```python
from build123d import *

# Parameters (mm, degrees)
F1_DEPTH = 200
F2_R     = 2
F4_DEPTH = 2


with BuildPart() as f1:
    # F0 (on Front) → F1 (new body)
    with BuildSketch(Plane.XZ):
        Polygon((35, 0), (0, 0), (0, -345), (28, -345), (28, -295), (8, -271.164928), (8, -191.164928), (30, -130.720425), (30, -80.720425), (28, -80.720425), (28, -130.367771), (6, -190.812274), (6, -271.892869), (26, -295.72794), (26, -343), (2, -343), (2, -2), (33, -2), (33, -23), (35, -23), align=None)
    extrude(amount=F1_DEPTH)

    # F2
    f2_edges = [f1.edges().sort_by_distance(p)[0] for p in [
        (0, -100, 0),
        (35, -100, 0),
        (33, -100, -2),
        (2, -100, -2),
        (0, -100, -345),
        (2, -100, -343),
        (28, -100, -345),
        (26, -100, -343),
        (26, -100, -295.72794),
        (28, -100, -295),
        (8, -100, -271.164928),
        (6, -100, -271.892869),
        (6, -100, -190.812274),
        (8, -100, -191.164928),
        (30, -100, -130.720425),
        (28, -100, -130.367771),
    ]]
    fillet(f2_edges, radius=F2_R)

    # F3 (on face) → F4 (cut)
    with BuildSketch(Plane(origin=(0, 0, 0), x_dir=(0, -1, 0), z_dir=(-1, 0, 0))):
        with BuildLine():
            Line((70, -50), (30, -50))
            ThreePointArc((30, -50), (26.464466, -51.464466), (25, -55))
            Line((25, -55), (25, -290))
            ThreePointArc((25, -290), (26.464466, -293.535534), (30, -295))
            Line((30, -295), (70, -295))
            ThreePointArc((70, -295), (73.535534, -293.535534), (75, -290))
            Line((75, -290), (75, -55))
            ThreePointArc((75, -55), (73.535534, -51.464466), (70, -50))
        make_face()
        with BuildLine():
            ThreePointArc((175, -55), (173.535534, -51.464466), (170, -50))
            Line((170, -50), (130, -50))
            ThreePointArc((130, -50), (126.464466, -51.464466), (125, -55))
            Line((125, -55), (125, -290))
            ThreePointArc((125, -290), (126.464466, -293.535534), (130, -295))
            Line((130, -295), (170, -295))
            ThreePointArc((170, -295), (173.535534, -293.535534), (175, -290))
            Line((175, -290), (175, -55))
        make_face()
    extrude(amount=-F4_DEPTH, mode=Mode.SUBTRACT)


solid = f1.part
```
Source: CAD feature listing. Evaluate the final solid. Frame: model axes, mm. A direction names the side the tool comes from. Give positions to 0.01 mm unless a question says otherwise; leave off trailing zeros. Order: outer loops, then holes, each group sorted by start corner. A loop starts at its lowest first (then second) coordinate and runs counter-clockwise, first axis right, second up. Notation, with made-up numbers: (-37.5, -13) -> (14.5, -13) arc R37 ccw to (14.5, 24) -> close; hole circle Ø8 at (76.5, 9). An arc over 180 degrees is marked (long way). Use a Markdown table: item, result.
Q1. Section A-A (z = -205). Return the cut outline in (x, y), and give its area (3 significant figures).
A:
| item | result |
|---|---|
| outline | (0, -200) -> (2, -200) -> (2, -175) -> (0, -175) -> close; (0, -125) -> (2, -125) -> (2, -75) -> (0, -75) -> close; (0, -25) -> (2, -25) -> (2, 0) -> (0, 0) -> close; (6, -200) -> (8, -200) -> (8, 0) -> (6, 0) -> close |
| area | 600 mm^2 |
Q2. Material intervals for line 1 (X direction, y = -166, z = -14.5); line 2 (X direction, y = -159, z = -191.5); line 3 (Z direction, x = 3.5, y = -19), sorted ascending. Write a range as [from, to].
A:
| item | result |
|---|---|
| line 1 | [0, 2], [33, 35] |
| line 2 | [6, 8] |
| line 3 | [-345, -342.94], [-2.06, 0] |
Q3. Pull-direction query (X, two-part tool) for faces 1 (the face through (0, -99, -170)), 2 (the face through (26, -99, -318)), 3 (the face through (14, -99, -345)); classes: +X half, -X half, draft (parallel to the pull), parting line (faces both ways), or undercut.
A:
| item | result |
|---|---|
| face 1 | -X half |
| face 2 | undercut |
| face 3 | draft |
Q4. First-contact query: P1, Ø1.6, axis at x = 1, y = -50, coming from the +Z side; P2, Ø1, axis at x = 1, y = -145, coming from the -Z side; P3, Ø4, axis at x = 4.5, z = -158, coming from the +Y side; P4, Ø23.5, axis at y = -84, z = -318, coming from the +X side. Flat tips, straight axial feed; report the tip coordinate or a pass-through.
A:
| item | result |
|---|---|
| P1 | z = -0.01 |
| P2 | z = -344.94 |
| P3 | through |
| P4 | x = 28 |
Q5. Section B-B (x = 15.5). Return the cut outline in (y, z), and give its area (3 significant figures).
A:
| item | result |
|---|---|
| outline | (-200, -345) -> (0, -345) -> (0, -343) -> (-200, -343) -> close; (-200, -283.21) -> (0, -283.21) -> (0, -280.1) -> (-200, -280.1) -> close; (-200, -170.56) -> (0, -170.56) -> (0, -164.71) -> (-200, -164.71) -> close; (-200, -2) -> (0, -2) -> (0, 0) -> (-200, 0) -> close |
| area | 2,590 mm^2 |
Q6. Access query for faces 4 (the face through (18.1, -98.6, -283.2)), 5 (the face through (33, -99, -13)), 6 (the face through (30, -99, -106)), 7 (the face through (14, -99, -343)). Directions: +Z, -Z, +X, -X, +Y, -Y. A direction counts if a zero-diameter tool reaches every point of the face in a straight line with its end or side. Return the directions, or none.
A:
| item | result |
|---|---|
| face 4 | +X, +Y, -Y |
| face 5 | -Z, +Y, -Y |
| face 6 | -Z, +X, +Y, -Y |
| face 7 | +Y, -Y |
